Here's how the part is built. I have some questions about the finished solid (model axes, mm). A direction names the side the tool comes from. Coordinates: 2 decimals unless noted, no trailing zeros. Write each loop counter-clockwise with the first axis right and the second up, starting at its lowest first coordinate (ties: lowest second). Pieces come first, ordered by that corner, then holes.
(1) Imagine slicing it at A-A, the plane z = 15.4. List the corners of the cut face in (x, y) for me, plus the area to 3 significant figures.
(2) For pin 1 Ø2 at (x, z) = (18.5, 18.5) entering from +Y; pin 2 Ø1.5 at (x, z) = (15.4, -15.4) entering from +Y; pin 3 Ø2.5 at (x, z) = (0, 2) entering from -Y, each with a flat end and sliding along its axis, tell me the tip position at first contact or that it passes through.
(3) Imagine slicing it at D-D, the plane z = 5.5. List the corners of the cut face in (x, y) for me, plus the area to 3 significant figures.
(4) Imagine slicing it at B-B, the plane x = -15.4. List the corners of the cut face in (y, z) for me.
(5) Please list where these lines run through material, in increasing order: probe 1 along Z at (x, y) = (-15.4, 34); probe 2 along Y at (x, z) = (-7.5, -16); probe 3 along X at (y, z) = (34, 15).
(6) Which directions (+Z, -Z, +X, -X, +Y, -Y) give clear straight access to the entire face, cutting with the end or side of a thin tool? Please do faces 1 (the flat face through (-18, 12, -18)), 2 (the flat face through (-18, 29, 18)), 3 (the flat face through (17.4, 20.4, -17.4)), 4 (the flat face through (-15, 29.6, 15)), 5 (the flat face through (17.4, 20.4, 17.4)).
(7) Imagine slicing it at C-C, the plane y = 45.5. List the corners of the cut face in (x, z) for me.
(8) Thinking about a two-plate mould opening in Z: for faces 6 (the cylindrical face through (15.977, 33.656, -14.291)), 7 (the flat face through (-18, 12, 18)), 8 (the cylindrical face through (-0.54, 47, 2.44)), which applies, released by +Z, released by -Z, zero draft, split by the parting line, or undercut?
```python
from build123d import *

# Parameters (mm, degrees)
SKETCH1_W               = 41.6
SKETCH1_H               = 41.6
BOSS_EXTRUDE1_DEPTH     = 37.6
SKETCH2_R               = 11
BOSS_EXTRUDE2_DEPTH     = 2.5
SKETCH3_R               = 2.5
BOSS_EXTRUDE3_DEPTH     = 14
SKETCH4_R               = 1.25
CUT_EXTRUDE1_DEPTH      = 8
MIRROR2_COPY_1_SKETCH_R = 1.25
MIRROR2_COPY_1_DEPTH    = 8
CUT_EXTRUDE2_DEPTH      = 17
MIRROR4_COPY_1_DEPTH    = 17
SKETCH10_R              = 4.3
CUT_EXTRUDE3_DEPTH      = 5.7


with BuildPart() as part:
    # Sketch1 → Boss-Extrude1 (new body)
    with BuildSketch(Plane(origin=(0, 0, 0), x_dir=(1, 0, 0), z_dir=(0, 1, 0))):
        Rectangle(SKETCH1_W, SKETCH1_H)
    extrude(amount=BOSS_EXTRUDE1_DEPTH)

    # Sketch2 → Boss-Extrude2 (add)
    with BuildSketch(Plane(origin=(0, 37.6, 0), x_dir=(1, 0, 0), z_dir=(0, 1, 0))):
        Circle(SKETCH2_R)
    extrude(amount=BOSS_EXTRUDE2_DEPTH)

    # Sketch3 → Boss-Extrude3 (add)
    with BuildSketch(Plane(origin=(0, 40.1, 0), x_dir=(1, 0, 0), z_dir=(0, 1, 0))):
        Circle(SKETCH3_R)
    extrude(amount=BOSS_EXTRUDE3_DEPTH)

    # Sketch4 → Cut-Extrude1 (cut)
    with BuildSketch(Plane(origin=(0, 37.6, 0), x_dir=(1, 0, 0), z_dir=(0, 1, 0))):
        with Locations((15.4, 15.4)):
            Circle(SKETCH4_R)
    cut_extrude1 = extrude(amount=-CUT_EXTRUDE1_DEPTH, mode=Mode.SUBTRACT)

    # Mirror1: Cut-Extrude1 across plane
    add(cut_extrude1.mirror(Plane(origin=(0, 0, 0), x_dir=(0, 0, 1), z_dir=(1, 0, 0))), mode=Mode.SUBTRACT)

    # Mirror2: Cut-Extrude1 across plane
    add(cut_extrude1.mirror(Plane.XY), mode=Mode.SUBTRACT)

    # Mirror2 copy 1 sketch → Mirror2 copy 1 (cut)
    with BuildSketch(Plane(origin=(0, 37.6, 0), x_dir=(-1, 0, 0), z_dir=(0, 1, 0))):
        with Locations((15.4, 15.4)):
            Circle(MIRROR2_COPY_1_SKETCH_R)
    extrude(amount=-MIRROR2_COPY_1_DEPTH, mode=Mode.SUBTRACT)

    # Sketch9 → Cut-Extrude2 (cut)
    with BuildSketch(Plane(origin=(0, 12, 0), x_dir=(1, 0, 0), z_dir=(0, 1, 0))):
        Polygon((20.8, 14), (14, 20.8), (20.8, 20.8), align=None)
    cut_extrude2 = extrude(amount=CUT_EXTRUDE2_DEPTH, mode=Mode.SUBTRACT)

    # Mirror3: Cut-Extrude2 across plane
    add(cut_extrude2.mirror(Plane.XY), mode=Mode.SUBTRACT)

    # Mirror4: Cut-Extrude2 across plane
    add(cut_extrude2.mirror(Plane(origin=(0, 0, 0), x_dir=(0, 0, 1), z_dir=(1, 0, 0))), mode=Mode.SUBTRACT)

    # Mirror4 copy 1 sketch → Mirror4 copy 1 (cut)
    with BuildSketch(Plane(origin=(0, 12, 0), x_dir=(-1, 0, 0), z_dir=(0, 1, 0))):
        Polygon((20.8, 14), (14, 20.8), (20.8, 20.8), align=None)
    extrude(amount=MIRROR4_COPY_1_DEPTH, mode=Mode.SUBTRACT)

    # Sketch10 → Cut-Extrude3 (cut)
    with BuildSketch(Plane.XZ):
        Circle(SKETCH10_R)
    extrude(amount=-CUT_EXTRUDE3_DEPTH, mode=Mode.SUBTRACT)


solid = part.part
```
Recorded:
1. outline: (-20.8, 0) - (20.8, 0) - (20.8, 12) - (19.4, 12) - (19.4, 29) - (20.8, 29) - (20.8, 37.6) - (16.65, 37.6) - (16.65, 29.6) - (14.15, 29.6) - (14.15, 37.6) - (-14.15, 37.6) - (-14.15, 29.6) - (-16.65, 29.6) - (-16.65, 37.6) - (-20.8, 37.6) - (-20.8, 29) - (-19.4, 29) - (-19.4, 12) - (-20.8, 12) - close
1. area: 1,480 mm2
2. pin 1: stops at y = 37.6
2. pin 2: stops at y = 29.6
2. pin 3: stops at y = 5.7
3. outline: (-20.8, 0) - (20.8, 0) - (20.8, 37.6) - (9.53, 37.6) - (9.53, 40.1) - (-9.53, 40.1) - (-9.53, 37.6) - (-20.8, 37.6) - close
3. area: 1,610 mm2
4. outline: (0, -20.8) - (12, -20.8) - (12, -19.4) - (29, -19.4) - (29, -20.8) - (37.6, -20.8) - (37.6, -16.65) - (29.6, -16.65) - (29.6, -14.15) - (37.6, -14.15) - (37.6, 14.15) - (29.6, 14.15) - (29.6, 16.65) - (37.6, 16.65) - (37.6, 20.8) - (29, 20.8) - (29, 19.4) - (12, 19.4) - (12, 20.8) - (0, 20.8) - close
5. probe 1: z = -20.8 to -16.65, -14.15 to 14.15, 16.65 to 20.8
5. probe 2: y = 0 to 37.6
5. probe 3: x = -20.8 to -16.58, -14.22 to 14.22, 16.58 to 20.8
6. face 1: -Z, -X
6. face 2: +Z, -X
6. face 3: -Z, +X
6. face 4: +Y
6. face 5: +Z, +X
7. outline: circle Ø5 at (0, 0)
8. face 6: undercut
8. face 7: zero draft
8. face 8: split by the parting line
